```python
from build123d import *

# Parameters (mm, degrees)
F0_R     = 10
F1_DEPTH = 3
F2_R     = 13.75
F3_DEPTH = 1
F4_R     = 0.99999


# Not quite as in the source:
# - a fillet or chamfer is up to 0.001 mm smaller than in the source, because OpenCascade refuses the exact size


with BuildPart() as f1:
    # F0 (on Front) → F1 (new body)
    with BuildSketch(Plane.XZ):
        with BuildLine():
            ThreePointArc((-7.0762930266, 10.0230719262), (-7.391479251, 8.3623594503), (-8.2420141709, 6.901572459))
            ThreePointArc((-8.2420141709, 6.901572459), (-9.3097730907, 5.375), (-10.097944161, 3.6870074208))
            ThreePointArc((-10.097944161, 3.6870074208), (-10.937755345, 2.2200290777), (-12.2183814254, 1.1167135625))
            ThreePointArc((-12.2183814254, 1.1167135625), (-12.85, 0), (-12.2183814254, -1.1167135625))
            ThreePointArc((-12.2183814254, -1.1167135625), (-10.937755345, -2.2200290777), (-10.097944161, -3.6870074208))
            ThreePointArc((-10.097944161, -3.6870074208), (-9.3097730907, -5.375), (-8.2420141709, -6.901572459))
            ThreePointArc((-8.2420141709, -6.901572459), (-7.391479251, -8.3623594503), (-7.0762930266, -10.0230719262))
            ThreePointArc((-7.0762930266, -10.0230719262), (-6.425, -11.1284264386), (-5.1420883988, -11.1397854887))
            ThreePointArc((-5.1420883988, -11.1397854887), (-3.5462760941, -10.582388528), (-1.8559299902, -10.5885798798))
            ThreePointArc((-1.8559299902, -10.5885798798), (0, -10.75), (1.8559299902, -10.5885798798))
            ThreePointArc((1.8559299902, -10.5885798798), (3.5462760941, -10.582388528), (5.1420883988, -11.1397854887))
            ThreePointArc((5.1420883988, -11.1397854887), (6.425, -11.1284264386), (7.0762930266, -10.0230719262))
            ThreePointArc((7.0762930266, -10.0230719262), (7.391479251, -8.3623594503), (8.2420141709, -6.901572459))
            ThreePointArc((8.2420141709, -6.901572459), (9.3097730907, -5.375), (10.097944161, -3.6870074208))
            ThreePointArc((10.097944161, -3.6870074208), (10.937755345, -2.2200290777), (12.2183814254, -1.1167135625))
            ThreePointArc((12.2183814254, -1.1167135625), (12.85, 0), (12.2183814254, 1.1167135625))
            ThreePointArc((12.2183814254, 1.1167135625), (10.937755345, 2.2200290777), (10.097944161, 3.6870074208))
            ThreePointArc((10.097944161, 3.6870074208), (9.3097730907, 5.375), (8.2420141709, 6.901572459))
            ThreePointArc((8.2420141709, 6.901572459), (7.391479251, 8.3623594503), (7.0762930266, 10.0230719262))
            ThreePointArc((7.0762930266, 10.0230719262), (6.425, 11.1284264386), (5.1420883988, 11.1397854887))
            ThreePointArc((5.1420883988, 11.1397854887), (3.5462760941, 10.582388528), (1.8559299902, 10.5885798798))
            ThreePointArc((1.8559299902, 10.5885798798), (0, 10.75), (-1.8559299902, 10.5885798798))
            ThreePointArc((-1.8559299902, 10.5885798798), (-3.5462760941, 10.582388528), (-5.1420883988, 11.1397854887))
            ThreePointArc((-5.1420883988, 11.1397854887), (-6.425, 11.1284264386), (-7.0762930266, 10.0230719262))
        make_face()
        Circle(F0_R, mode=Mode.SUBTRACT)
    extrude(amount=F1_DEPTH)

    # F2 (on Front) → F3 (join)
    with BuildSketch(Plane.XZ):
        Circle(F2_R)
    extrude(amount=-F3_DEPTH)

    # F4 (radius 1 in the source; OpenCascade refuses exactly that, so slightly less here)
    f4_edges = [f1.edges().sort_by_distance(p)[0] for p in [
        (-13.75, 1, 0),
    ]]
    fillet(f4_edges, radius=F4_R)


solid = f1.part
```
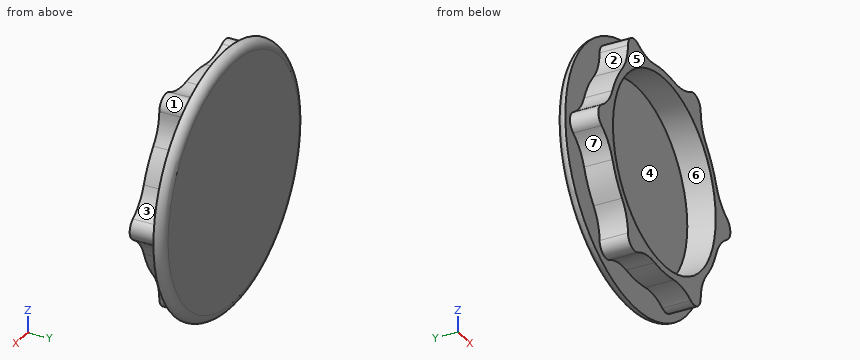
Geometry check sheet. Reference: the model listing, model coordinates, mm. Face numbers are marked on the shaded views. A direction names the side the tool comes from. Coordinates: 2 decimals unless noted, no trailing zeros. Order: outer loops, then holes, each group sorted by start corner. A loop starts at its lowest first (then second) coordinate and runs counter-clockwise, first axis right, second up. Notation, with made-up numbers: (-13.5, 41.5) - (16.5, 41.5) arc R34 cw to (16.5, 71.5) - close; hole circle Ø8 at (-5, -20). An arc over 180 degrees is marked (long way). Answer in a Markdown table with one row per item. Add a question column.
1. Material ranges on L1, parallel to Z at x = 0, y = -1.35; L2, parallel to Y at x = 3.75, z = 9; L3, parallel to X at y = -2.4, z = -11, recorded low to high. Write a range as [from, to].
2. Draft check along Z on the marked faces 4, 5, 6 and 7. Enter one of: +Z half, -Z half, draft (parallel to the pull), parting line (faces both ways), or undercut.
3. Gauge pin test, flat ends, axial feed: pin 1 Ø1.5 at (y, z) = (-1, 7.5) entering from -X; pin 2 Ø16 at (x, z) = (3, 0) entering from -Y. Record the tip position at first contact, or that the pin passes through.
4. Access from +Z, -Z, +X, -X, +Y, -Y to the whole of each face (thin tool, end or side, straight path). Record for the marked faces 1, 2 and 3.
5. Section check C-C (y = -0.5). Enter the section's corners in (x, z), plus the area to 3 significant figures.
Data:
| question | item | result |
|---|---|---|
| 1 | L1 | z = [-10.75, -10], [10, 10.75] |
| 1 | L2 | y = [0, 1] |
| 1 | L3 | x = [-6.61, -4.87], [4.87, 6.61] |
| 2 | face 4 | undercut |
| 2 | face 5 | draft |
| 2 | face 6 | undercut |
| 2 | face 7 | -Z half |
| 3 | pin 1 | stops at x = -8.37 |
| 3 | pin 2 | stops at y = -3 |
| 4 | face 1 | +Z, -Y |
| 4 | face 2 | +Z, -X, -Y |
| 4 | face 3 | +Z, +X, -Y |
| 5 | outline | (-12.22, -1.12) arc R5 cw to (-10.1, -3.69) arc R10.75 ccw to (-8.24, -6.9) arc R5 cw to (-7.08, -10.02) arc R1.3 ccw to (-5.14, -11.14) arc R5 cw to (-1.86, -10.59) arc R10.75 ccw to (1.86, -10.59) arc R5 cw to (5.14, -11.14) arc R1.3 ccw to (7.08, -10.02) arc R5 cw to (8.24, -6.9) arc R10.75 ccw to (10.1, -3.69) arc R5 cw to (12.22, -1.12) arc R1.3 ccw to (12.22, 1.12) arc R5 cw to (10.1, 3.69) arc R10.75 ccw to (8.24, 6.9) arc R5 cw to (7.08, 10.02) arc R1.3 ccw to (5.14, 11.14) arc R5 cw to (1.86, 10.59) arc R10.75 ccw to (-1.86, 10.59) arc R5 cw to (-5.14, 11.14) arc R1.3 ccw to (-7.08, 10.02) arc R5 cw to (-8.24, 6.9) arc R10.75 ccw to (-10.1, 3.69) arc R5 cw to (-12.22, 1.12) arc R1.3 ccw to start; hole circle Ø20 at (0, 0) |
| 5 | area | 89.0 mm² |
